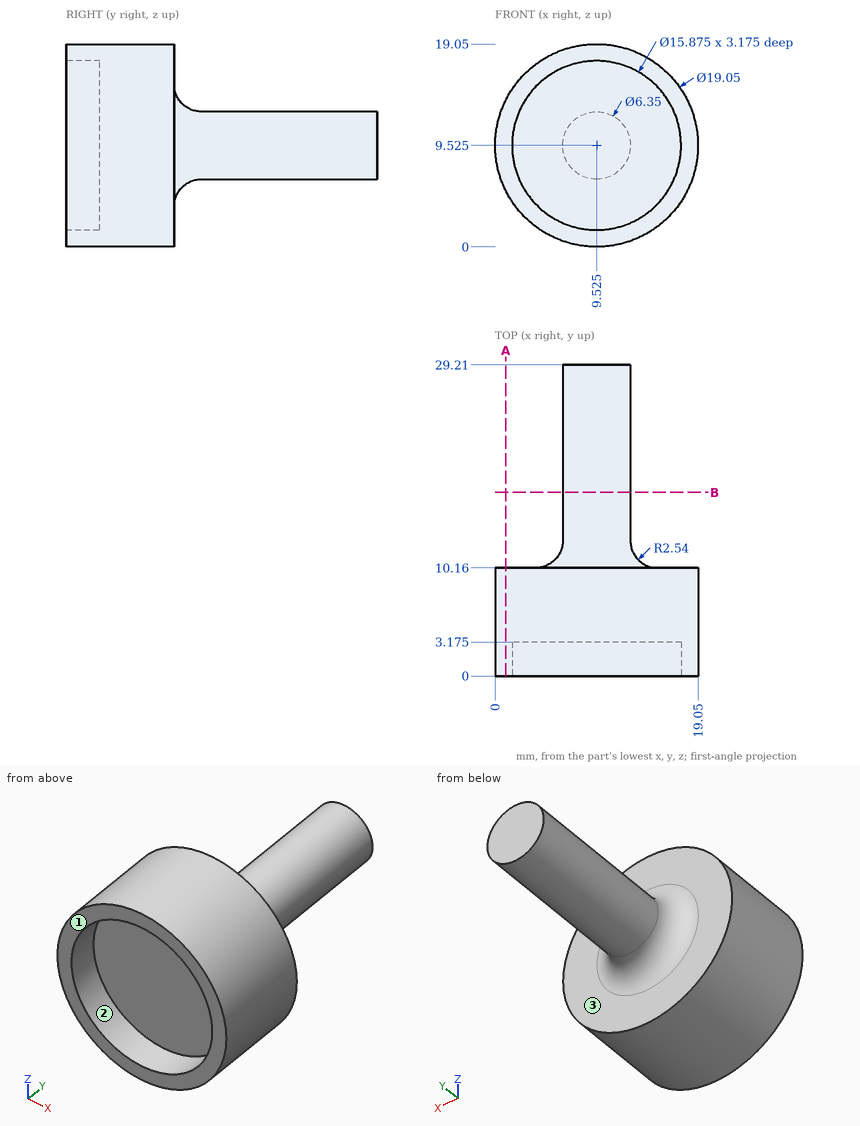
Check sheet for the drawn part. Datum: minimum x, y, z corner. Units: mm. A direction names the side the tool comes from. Coordinates: 2 decimals unless noted, no trailing zeros. Order: outer loops, then holes, each group sorted by start corner. A loop starts at its lowest first (then second) coordinate and runs counter-clockwise, first axis right, second up. Notation, with made-up numbers: M 51,-23.5 L 72,-23.5 A35 cw 72,8.5 Z; hole C 55,43.5 d2. An arc over 180 degrees is marked long. One line per item, written item: value. Start each with the question number.
Item 1: Scan lines: probe 1 along Y at (x, z) = (16.5, 13.25) (3 decimals); probe 2 along Y at (x, z) = (10.5, 12.5) (3 decimals); probe 3 along Z at (x, y) = (10.5, 1.5). Record each from-to range of solid material in increasing order.
Item 2: Sectioned sample at B-B (y = 17.25). Enter the section's corners in (x, z) (3 decimals).
Item 3: Sectioned sample at A-A (x = 1). Enter the section's corners in (y, z), then the cut area to 3 significant figures.
Item 4: Access from +Z, -Z, +X, -X, +Y, -Y to the whole of each face (thin tool, end or side, straight path). Record for the marked faces 1, 2 and 3.
Item 5: Gauge pin test, flat ends, axial feed: pin 1 (6 mm diameter, centred on y = 4.5, z = 5.5, fed in from -X); pin 2 (3 mm diameter, centred on x = 3.5, y = 3.5, fed in from +Z); pin 3 (2 mm diameter, centred on x = 16.5, y = 8, fed in from -Z). Record the tip position at first contact, or that the pin passes through.
Conclusion:
1. probe 1: y = 3.175 to 10.16
1. probe 2: y = 3.175 to 29.21
1. probe 3: z = 0.05 to 1.65, 17.4 to 19
2. outline: C 9.525,9.525 d6.35
3. outline: M 0,5.28 L 10.16,5.28 L 10.16,13.77 L 0,13.77 Z
3. area: 86.3 mm^2
4. face 1: +Z, -Z, +X, -X, -Y
4. face 2: -Y
4. face 3: +Y
5. pin 1: stops at x = 0.06
5. pin 2: stops at z = 17.91
5. pin 3: stops at z = 2.11
